Work out the finished part from the listing and answer in its coordinate system (mm). Give positions to 0.01 mm unless a question says otherwise; leave off trailing zeros. Write each loop counter-clockwise with the first axis right and the second up, starting at its lowest first coordinate (ties: lowest second). Pieces come first, ordered by that corner, then holes.
1) Straight lines are drawn through the part: probe 1 along Z at (x, y) = (-11, 770.5); probe 2 along Z at (x, y) = (-2.75, 538); probe 3 along X at (y, z) = (723, 19.75). For each, find the intervals that lie inside material, in ascending order.
2) Find section C-C (z = 18.75). Determine the outline of the cut face in (x, y), plus the area to 3 significant figures.
3) Given pin 1 Ø4 at (x, z) = (-9.5, 8.5) entering from +Y; pin 2 Ø6 at (y, z) = (960, 17.5) entering from +X; pin 3 Ø1 at (y, z) = (763.5, 4.5) entering from -X; pin 4 Ø1 at (y, z) = (913, 19) entering from -X, each flat-ended and moving along its own axis, determine where each tip first touches the part or whether it passes through.
4) Find section B-B (x = -11.5). Determine the outline of the cut face in (y, z), plus the area to 3 significant figures.
5) Find section A-A (y = 213). Determine the outline of the cut face in (x, z), plus the area to 3 significant figures.
Autodesk Inventor part; units mm, degrees
ref_plane "YZ Plane" through (0, 0, 0) normal (1, 0, 0) x (0, 1, 0)
ref_plane "XZ Plane" through (0, 0, 0) normal (0, 1, 0) x (-1, 0, 0)
ref_plane "XY Plane" through (0, 0, 0) normal (0, 0, 1) x (1, 0, 0)
sketch "Sketch1" plane through (0, 0, 0) normal (0, 1, 0) x (-1, 0, 0)
  line L0 (2.54, 0) -> (25.4, 0)
  line L1 (0, 25.4) -> (0, 2.54)
  line L2 (22.86, 4.7625) -> (7.3025, 4.7625)
  line L3 (4.7625, 7.3025) -> (4.7625, 22.86)
  line L4 (2.2225, 25.4) -> (0, 25.4)
  line L5 (25.4, 2.2225) -> (25.4, 0)
  arc A0 (4.7625, 7.3025) -> (7.3025, 4.7625) centre (7.3025, 7.3025) ccw
  arc A1 (4.7625, 22.86) -> (2.2225, 25.4) centre (2.2225, 22.86) ccw
  arc A2 (0, 2.54) -> (2.54, 0) centre (2.54, 2.54) ccw
  arc A3 (25.4, 2.2225) -> (22.86, 4.7625) centre (22.86, 2.2225) ccw
  point P0 (0, 0)
  dimension "d2" = 4.7625
  dimension "d3" = 25.4
  dimension "d4" = 25.4
  dimension "d5" = 2.54
extrude "Angle Iron Template" add sketch "Sketch1" along normal blind 1828.8
properties part number "legs-f_t"
Results:
1. probe 1: z = 0 to 4.76
1. probe 2: z = 0 to 25.34
1. probe 3: x = -4.76 to 0
2. outline: (-4.76, 0) - (0, 0) - (0, 1828.8) - (-4.76, 1828.8) - close
2. area: 8,710 mm2
3. pin 1: passes through
3. pin 2: stops at x = 0
3. pin 3: stops at x = -24.67
3. pin 4: stops at x = -4.76
4. outline: (0, 0) - (1828.8, 0) - (1828.8, 4.76) - (0, 4.76) - close
4. area: 8,710 mm2
5. outline: (-25.4, 0) - (-2.54, 0) arc R2.54 ccw to (0, 2.54) - (0, 25.4) - (-2.22, 25.4) arc R2.54 ccw to (-4.76, 22.86) - (-4.76, 7.3) arc R2.54 cw to (-7.3, 4.76) - (-22.86, 4.76) arc R2.54 ccw to (-25.4, 2.22) - close
5. area: 216 mm2
